from build123d import *

# Parameters (mm, degrees)
SKETCH1_W           = 7.14375
SKETCH1_H           = 5.159375
BOSS_EXTRUDE1_DEPTH = 14.2875
SKETCH1_3_W         = 19.161125
SKETCH1_3_H         = 7
BOSS_EXTRUDE2_DEPTH = 10
BOSS_EXTRUDE3_DEPTH = 1.5875
SKETCH1_5_R         = 1.190625
CUT_EXTRUDE1_DEPTH  = 1.5875
SKETCH2_R           = 4.7625
BOSS_EXTRUDE4_DEPTH = 11.1125
SKETCH2_3_R         = 3.175
BOSS_EXTRUDE5_DEPTH = 4.7625


with BuildPart() as part:
    # Sketch1 → Boss-Extrude1 (new body)
    with BuildSketch(Plane(origin=(0, 0, 0), x_dir=(1, 0, 0), z_dir=(0, 1, 0))):
        with Locations((-4.7625, 34.3296875)):
            Rectangle(SKETCH1_W, SKETCH1_H)
    extrude(amount=BOSS_EXTRUDE1_DEPTH)



with BuildPart() as body_2:
    # Sketch1_3 → Boss-Extrude2 (new body)
    with BuildSketch(Plane(origin=(0, 0, 0), x_dir=(1, 0, 0), z_dir=(0, 1, 0))):
        with Locations((1.1350625, -31.6)):
            Rectangle(SKETCH1_3_W, SKETCH1_3_H)
    extrude(amount=BOSS_EXTRUDE2_DEPTH)


with BuildPart() as part_1:
    add(part.part)

    add(body_2.part)  # Boss-Extrude3 merges body 2
    # Sketch1_4 → Boss-Extrude3 (add)
    with BuildSketch(Plane(origin=(0, 0, 0), x_dir=(1, 0, 0), z_dir=(0, 1, 0))):
        with BuildLine():
            Line((18.494375, -38.1), (-18.494375, -38.1))
            ThreePointArc((-18.494375, -38.1), (-20.290426224, -37.356051224), (-21.034375, -35.56))
            Line((-21.034375, -35.56), (-21.034375, 35.56))
            ThreePointArc((-21.034375, 35.56), (-20.290426224, 37.356051224), (-18.494375, 38.1))
            Line((-18.494375, 38.1), (18.494375, 38.1))
            ThreePointArc((18.494375, 38.1), (20.290426224, 37.356051224), (21.034375, 35.56))
            Line((21.034375, 35.56), (21.034375, -35.56))
            ThreePointArc((21.034375, -35.56), (20.290426224, -37.356051224), (18.494375, -38.1))
        make_face()
    extrude(amount=-BOSS_EXTRUDE3_DEPTH)

    # Sketch1_5 → Cut-Extrude1 (cut)
    with BuildSketch(Plane(origin=(0, 0, 0), x_dir=(1, 0, 0), z_dir=(0, 1, 0))):
        with Locations(Location((-17.4625, 34.528125, 0), (0, 0, 270))):
            Circle(SKETCH1_5_R)
        with Locations(Location((-17.4625, -34.528125, 0), (0, 0, 270))):
            Circle(SKETCH1_5_R)
        with Locations(Location((17.4625, -34.528125, 0), (0, 0, 270))):
            Circle(SKETCH1_5_R)
        with Locations(Location((17.4625, 34.528125, 0), (0, 0, 90))):
            Circle(SKETCH1_5_R)
    extrude(amount=-CUT_EXTRUDE1_DEPTH, mode=Mode.SUBTRACT)

    # Sketch2 → Boss-Extrude4 (add)
    with BuildSketch(Plane(origin=(0, 0, 0), x_dir=(1, 0, 0), z_dir=(0, 1, 0))):
        with Locations(Location((-14.684375, -25.4, 0), (0, 0, 90))):
            Circle(SKETCH2_R)
    extrude(amount=BOSS_EXTRUDE4_DEPTH)

    # Sketch2_3 → Boss-Extrude5 (add)
    with BuildSketch(Plane(origin=(0, 0, 0), x_dir=(1, 0, 0), z_dir=(0, 1, 0))):
        with Locations(Location((-15.954375, -6.35, 0), (0, 0, 90))):
            Circle(SKETCH2_3_R)
        with Locations(Location((-8.334375, 12.7, 0), (0, 0, 90))):
            Circle(SKETCH2_3_R)
    extrude(amount=BOSS_EXTRUDE5_DEPTH)


solid = part_1.part
Check sheet for the modelled part. Datum: model origin and axes. Units: mm. A direction names the side the tool comes from. Round coordinates to 2 decimals unless told otherwise and drop trailing zeros. Order: outer loops, then holes, each group sorted by start corner. A loop starts at its lowest first (then second) coordinate and runs counter-clockwise, first axis right, second up.
Q1. Cross-section at D-D, the plane y = 12.5. Enter the section's corners in (x, z), plus the area to 3 significant figures.
Filled sheet:
outline: (-8.33, -36.91) - (-1.19, -36.91) - (-1.19, -31.75) - (-8.33, -31.75) - close
area: 36.9 mm2
Q2. Cross-section at C-C, the plane y = 3.25. Give the number of separate pieces and of enclosed holes in the cut face, plus the area to 3 significant figures.
Filled sheet:
separate pieces: 5
enclosed holes: 0
area: 306 mm2
Q3. Depth check by flat-ended pin: P1, Ø12, axis at x = 14.5, z = -5.5, coming from the +Y side; P2, Ø2.5, axis at y = 5, z = -35.5, coming from the -X side; P3, Ø3, axis at x = -16.5, z = 6.5, coming from the +Y side; P4, Ø2, axis at x = -17.46, z = 34.53, coming from the +Y side. Enter the tip coordinate at first touch or a pass-through.
Filled sheet:
P1: stops at y = 0
P2: stops at x = -8.33
P3: stops at y = 4.76
P4: passes through
Q4. Scan lines: L1, parallel to Z at x = -4, y = 6.75; L2, parallel to Y at x = -10, z = 18; L3, parallel to Z at x = 4.5, y = 4.5. Record each from-to range of solid material in increasing order.
Filled sheet:
L1: z = -36.91 to -31.75, 28.1 to 35.1
L2: y = -1.59 to 0
L3: z = 28.1 to 35.1
Q5. Cross-section at A-A, the plane x = 2.5. Enter the section's corners in (y, z), plus the area to 3 significant figures.
Filled sheet:
outline: (-1.59, -38.1) - (0, -38.1) - (0, 28.1) - (10, 28.1) - (10, 35.1) - (0, 35.1) - (0, 38.1) - (-1.59, 38.1) - close
area: 191 mm2
Q6. Cross-section at B-B, the plane z = 25.4. Enter the section's corners in (x, y).
Filled sheet:
outline: (-21.03, -1.59) - (21.03, -1.59) - (21.03, 0) - (-9.92, 0) - (-9.92, 11.11) - (-19.45, 11.11) - (-19.45, 0) - (-21.03, 0) - close
Q7. Set-up check for faces 5 (the face through (-5, 7, -31.75)), 6 (the face through (10.716, 5, 32)), 7 (the face through (-16.115, 5.478, 20.857)): record each of +Z, -Z, +X, -X, +Y, -Y from which the full face is reachable in a straight line by a thin tool's end or side.
Filled sheet:
face 5: +X, -X, +Y
face 6: +Z, -Z, +X, +Y
face 7: +Y
Q8. Draft check along X on faces 1 (the face through (-20.31, -0.783, -37.336)), 2 (the face through (0, -1, -38.1)), 3 (the face through (17.919, -0.783, -35.628)), 4 (the face through (21.034, -1, 0)). Enter one of: pulls with the +X half, pulls with the -X half, needs draft (parallel to the pull), parting line crosses it, or undercut.
Filled sheet:
face 1: pulls with the -X half
face 2: needs draft
face 3: undercut
face 4: pulls with the +X half
